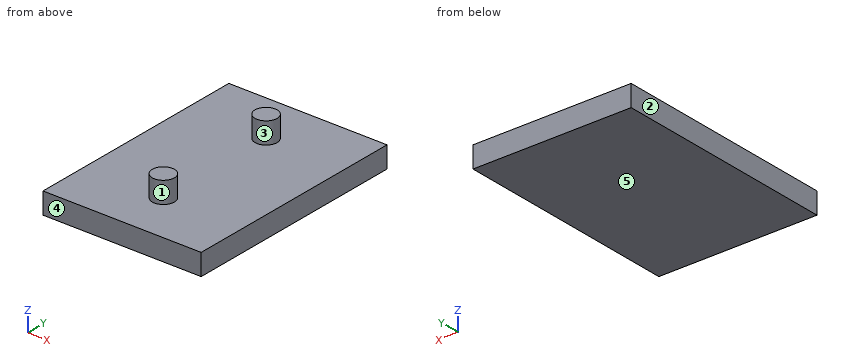
from build123d import *

# Parameters (mm, degrees)
F0_R     = 6.587006
F1_DEPTH = 12.7
F2_DEPTH = 25.4


with BuildPart() as f1:
    # F0 (on Top) → F1 (new body)
    with BuildSketch(Plane.XY):
        Polygon((0, 50.230512), (-47.195485, 50.230512), (-47.195485, 19.750512), (-47.195485, -54.646088), (-47.195485, -85.126088), (0, -85.126088), (47.195485, -85.126088), (47.195485, -54.646088), (47.195485, 19.750512), (47.195485, 50.230512), align=None)
        with Locations((0, -55.052097)):
            Circle(F0_R, mode=Mode.SUBTRACT)
        with Locations((0, 19.750512)):
            Circle(F0_R, mode=Mode.SUBTRACT)
        with Locations((0, 19.750512)):
            Circle(F0_R)
        with Locations((0, -55.052097)):
            Circle(F0_R)
    extrude(amount=F1_DEPTH)

    # F0 (on Top) → F2 (join)
    with BuildSketch(Plane.XY):
        with Locations((0, 19.750512)):
            Circle(F0_R)
        with Locations((0, -55.052097)):
            Circle(F0_R)
    extrude(amount=F2_DEPTH)


solid = f1.part
Design review of the part built by this model. Coordinates are the model's own, in mm. Face numbers are marked on the shaded views. A direction names the side the tool comes from. Round coordinates to 2 decimals unless told otherwise and drop trailing zeros. Write each loop counter-clockwise with the first axis right and the second up, starting at its lowest first coordinate (ties: lowest second). Pieces come first, ordered by that corner, then holes.
Item 1: For the marked faces 1 and 2, list the 3-axis set-ups (+Z, -Z, +X, -X, +Y, -Y) from which the entire face can be reached by the end or side of a thin tool; tool diameter is ignored.
Item 2: Draft analysis for pull direction Y (two halves, no side actions). For the marked faces 3, 4 and 5, state which applies: released by +Y, released by -Y, zero draft, split by the parting line, or undercut.
Item 3: Consider section B-B on y = -66. Give the boundary of the cut face in (x, z), and give its area (3 significant figures).
Item 4: Consider section A-A on x = 0. Give the boundary of the cut face in (y, z), and give its area (3 significant figures).
Item 5: Consider section C-C on x = 24. Give the boundary of the cut face in (y, z), and give its area (3 significant figures).
Item 6: Wall thickness on L1, parallel to Z at x = -24, y = -69: over which ranges is the line inside the solid? List them lowest first.
Item 7: For pin 1 Ø6 at (x, y) = (-30, 20.5) entering from -Z; pin 2 Ø12 at (x, z) = (-17, 20) entering from +Y; pin 3 Ø3 at (x, y) = (21, -15) entering from +Z, all flat-tipped, find the tip position at first contact; note any pin that passes through.
Check values:
1. face 1: +Z
1. face 2: +Z, -Z, -X, +Y, -Y
2. face 3: undercut
2. face 4: released by -Y
2. face 5: zero draft
3. outline: (-47.2, 0) - (47.2, 0) - (47.2, 12.7) - (-47.2, 12.7) - close
3. area: 1,200 mm2
4. outline: (-85.13, 0) - (50.23, 0) - (50.23, 12.7) - (26.34, 12.7) - (26.34, 25.4) - (13.16, 25.4) - (13.16, 12.7) - (-48.47, 12.7) - (-48.47, 25.4) - (-61.64, 25.4) - (-61.64, 12.7) - (-85.13, 12.7) - close
4. area: 2,050 mm2
5. outline: (-85.13, 0) - (50.23, 0) - (50.23, 12.7) - (-85.13, 12.7) - close
5. area: 1,720 mm2
6. L1: z = 0 to 12.7
7. pin 1: stops at z = 0
7. pin 2: passes through
7. pin 3: stops at z = 12.7
